For this review, take the finished solid that the model builds, in its own axes (mm). Round coordinates to 2 decimals unless told otherwise and drop trailing zeros. Write each loop counter-clockwise with the first axis right and the second up, starting at its lowest first coordinate (ties: lowest second). Pieces come first, ordered by that corner, then holes. Notation, with made-up numbers: (68.25, 31) -> (82.25, 31) arc R34 cw to (82.25, 68) -> close; hole circle Ø4 at (43, 60). An arc over 180 degrees is marked (long way). Answer in a Markdown table with one row per item.
from build123d import *

# Parameters (mm, degrees)
SKIZZE1_W                       = 2000
SKIZZE1_H                       = 800
AUFSATZ_LINEAR_AUSTRAGEN1_DEPTH = 16
SCHNITT_LINEAR_AUSTRAGEN1_DEPTH = 17


with BuildPart() as part:
    # Skizze1 → Aufsatz-Linear austragen1 (new body)
    with BuildSketch(Plane.XY):
        Rectangle(SKIZZE1_W, SKIZZE1_H)
    extrude(amount=AUFSATZ_LINEAR_AUSTRAGEN1_DEPTH)

    # Skizze2 → Schnitt-Linear austragen1 (cut, through all)
    with BuildSketch(Plane.XY.offset(16)):
        Polygon((-300, -400), (-300, 0), (-1381.908908696, 0), (-1381.908908696, -457.580605906), (-300, -457.580605906), align=None)
        Polygon((1381.908908696, -457.580605906), (300, -457.580605906), (300, -400), (300, 0), (1381.908908696, 0), align=None)
    extrude(amount=-SCHNITT_LINEAR_AUSTRAGEN1_DEPTH, mode=Mode.SUBTRACT)


solid = part.part
1) For line 1 (Y direction, x = 914.5, z = 4); line 2 (X direction, y = -99.5, z = 6.5), list the stretches that pass through material, from the lowest coordinate up. Write a range as [from, to].
Solved:
| item | result |
|---|---|
| line 1 | [0, 400] |
| line 2 | [-300, 300] |
2) Consider section C-C on y = -334.5. State the section outline as (x, z) points.
Solved:
| item | result |
|---|---|
| outline | (-300, 0) -> (300, 0) -> (300, 16) -> (-300, 16) -> close |
3) Consider section A-A on z = 8.5. State the section outline as (x, y) points.
Solved:
| item | result |
|---|---|
| outline | (-1000, 0) -> (-300, 0) -> (-300, -400) -> (300, -400) -> (300, 0) -> (1000, 0) -> (1000, 400) -> (-1000, 400) -> close |
4) Consider section B-B on x = 636.5. State the section outline as (y, z) points, then the cut area to 3 significant figures.
Solved:
| item | result |
|---|---|
| outline | (0, 0) -> (400, 0) -> (400, 16) -> (0, 16) -> close |
| area | 6,400 mm² |
5) Clearance check with flat-ended pins moving along their axes: pin 1 Ø5 at (x, z) = (-631.5, 11.5) entering from -Y; pin 2 Ø4 at (y, z) = (-153.5, 5) entering from +X. State where each tip first meets the part, or that it passes through.
Solved:
| item | result |
|---|---|
| pin 1 | y = 0 |
| pin 2 | x = 300 |
